Can you work these out from the model? Positions are in its coordinate system, mm. Round coordinates to 2 decimals unless told otherwise and drop trailing zeros. Write each loop counter-clockwise with the first axis right and the second up, starting at its lowest first coordinate (ties: lowest second). Pieces come first, ordered by that corner, then holes. Notation, with made-up numbers: M 38,-11 L 52,-11 A24 cw 52,2 Z; hole C 12.5,86.25 d7. An arc over 180 degrees is marked long. Answer in a Markdown table with one row per item. Add a question column.
(1) Suppose I cut it at A-A, the plane x = 0. Write out the boundary of the cut face in (y, z).
(2) If I drill on probe 1 along Z at (x, y) = (0, 20.5); probe 2 along Z at (x, y) = (16, 21.3); probe 3 along Z at (x, y) = (-2.5, 21.4), over which ranges is the centre line in solid material (lowest first)?
(3) Suppose I cut it at C-C, the plane z = 0. Write out the boundary of the cut face in (x, y), then the cut area to 3 significant figures.
(4) If we mould it in two halves opening along X, with no side actions, what happens to faces 1 (the face through (0, 22, -29)), 2 (the face through (-23.452, 20.479, -8.796)), 3 (the face through (-8.767, 20.479, 16.856)), 4 (the face through (0.408, 20.479, 21.246))? For each: released by +X, released by -X, zero draft, split by the parting line, or undercut.
(5) Suppose I cut it at D-D, the plane x = -11. Write out the boundary of the cut face in (y, z), then the cut area to 3 significant figures.
(6) Suppose I cut it at B-B, the plane z = -38.5. Write out the boundary of the cut face in (x, y), then the cut area to 3 significant figures.
Autodesk Inventor part; units mm, degrees
ref_plane "YZ Plane" through (0, 0, 0) normal (1, 0, 0) x (0, 1, 0)
ref_plane "XZ Plane" through (0, 0, 0) normal (0, 1, 0) x (-1, 0, 0)
ref_plane "XY Plane" through (0, 0, 0) normal (0, 0, 1) x (1, 0, 0)
sketch "Эскиз1" plane through (19.6324, 19, -8.132) normal (0, 1, 0) x (-1, 0, 0)
  circle A0 centre (19.6324, -30.368) radius 2
  line L0 (-6.3676, -13.3012) -> (45.6324, -13.3012)
  line L1 (45.6324, -13.3012) -> (45.6324, -40.368)
  line L2 (45.6324, -40.368) -> (-6.3676, -40.368)
  line L3 (-6.3676, -40.368) -> (-6.3676, -13.3012)
  circle A1 centre (35.6324, -30.368) radius 2
  circle A2 centre (3.6324, -30.368) radius 2
  circle A3 centre (19.6324, 8.132) radius 21.25
  line L4 (-6.3676, -13.3012) -> (-1.1982, 12.3327)
  line L5 (45.6324, -13.3012) -> (40.4631, 12.3327)
  circle A4 centre (19.6324, 8.132) radius 19
  point P0 (19.6324, -13.3012)
  dimension "d0" = 4
  dimension "d1" = 38.5
  dimension "d2" = 4
  dimension "d3" = 16
  dimension "d4" = 4
  dimension "d5" = 16
  dimension "d6" = 10
  dimension "d7" = 10
  dimension "d8" = 10
  dimension "d9" = 0
  dimension "d10" = 42.5
  dimension "d11" = 38
extrude "Выдавливание1" add sketch "Эскиз1" along normal blind 3
sketch "Эскиз2" plane through (20.8701, -13, -4) normal (0, 0, 1) x (1, 0, 0)
  line L0 (-44.8118, 9.5085) -> (8.0594, 9.5085)
  line L1 (8.0594, 9.5085) -> (8.0594, -14.2907)
  line L2 (8.0594, -14.2907) -> (-44.8118, -14.2907)
  line L3 (-44.8118, -14.2907) -> (-44.8118, 9.5085)
  point P0 (-20.8701, 13)
extrude "Выдавливание2" cut sketch "Эскиз2" along normal blind 30
sketch "Эскиз3" plane through (19.6324, 19, -8.132) normal (0, -1, 0) x (1, 0, 0)
  circle A0 centre (-19.6324, 8.132) radius 21.25
  dimension "d16" = 42.5
properties part number "Заднее крпление"
Calculated:
| question | item | result |
|---|---|---|
| 1 | outline | M 19,-48.5 L 22,-48.5 L 22,-40.5 L 19,-40.5 Z; M 19,-36.5 L 22,-36.5 L 22,-19 L 19,-19 Z; M 19,19 L 22,19 L 22,21.25 L 19,21.25 Z |
| 2 | probe 1 | -48.5 to -40.5, -36.5 to -19, 19 to 21.25 |
| 2 | probe 2 | -48.5 to -40.5, -36.5 to -10.25, 10.25 to 13.98 |
| 2 | probe 3 | -48.5 to -18.83, 18.83 to 21.1 |
| 3 | outline | M -21.68,19 L -19,19 L -19,22 L -21.68,22 Z; M 19,19 L 21.68,19 L 21.68,22 L 19,22 Z |
| 3 | area | 16.1 mm² |
| 4 | face 1 | zero draft |
| 4 | face 2 | released by -X |
| 4 | face 3 | undercut |
| 4 | face 4 | split by the parting line |
| 5 | outline | M 19,-48.5 L 22,-48.5 L 22,-15.49 L 19,-15.49 Z; M 19,15.49 L 22,15.49 L 22,18.18 L 19,18.18 Z |
| 5 | area | 107 mm² |
| 6 | outline | M -26,19 L -18,19 L -18,22 L -26,22 Z; M -14,19 L -2,19 L -2,22 L -14,22 Z; M 2,19 L 14,19 L 14,22 L 2,22 Z; M 18,19 L 26,19 L 26,22 L 18,22 Z |
| 6 | area | 120 mm² |
